Input: part model. Units: mm. Frame: model coordinates. Face numbers are marked on the shaded views. Give positions to 0.01 mm unless a question says otherwise; leave off trailing zeros. Write each loop counter-clockwise with the first axis right and the second up, starting at its lowest first coordinate (ties: lowest second). Pieces come first, ordered by that corner, then holes. Notation, with made-up numbers: (79, 29.25) - (112, 29.25) arc R25 ccw to (112, 42.25) - close; hole circle Ø2 at (-1.5, 19.5). An arc over 180 degrees is marked (long way). Use a Markdown table: item, result. Add a question column.
1. Section query D-D, the plane y = 6. Return loops of the section in (x, z), plus the area to 3 significant figures.
2. Section query B-B, the plane z = 0. Return loops of the section in (x, y), plus the area to 3 significant figures.
3. Mould query, pull axis Z, two halves, no side actions, for the marked faces 1, 2 and 3. Classes: released by +Z, released by -Z, zero draft, split by the parting line, or undercut.
4. Section query C-C, the plane x = 9.5. Return loops of the section in (y, z).
5. Pin query (flat end, axial travel): pin 1 (2 mm diameter, centred on x = -10, y = 8, fed in from -Z); pin 2 (2 mm diameter, centred on x = 2.5, y = 8.5, fed in from -Z); pin 3 (1.5 mm diameter, centred on y = 4, z = 8.5, fed in from -X). Return the tip coordinate at first contact, or that it passes through.
6. Section query A-A, the plane x = 0. Return loops of the section in (y, z), plus the area to 3 significant figures.
7. Material intervals for probe 1 along X at (y, z) = (6.25, 0); probe 2 along X at (y, z) = (8, 1); probe 3 along X at (y, z) = (2.25, 3), sorted ascending.
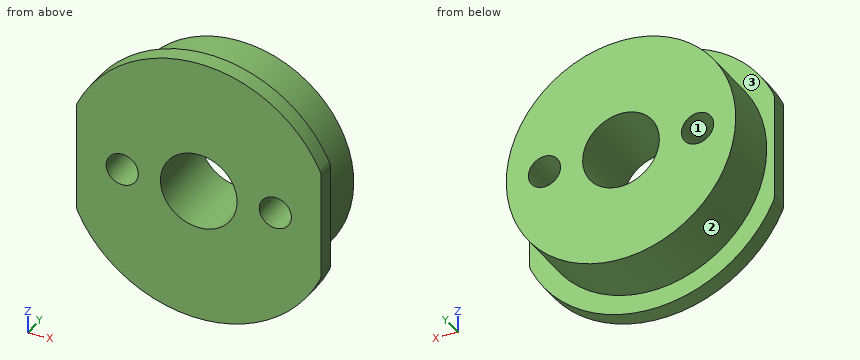
```python
from build123d import *

# Parameters (mm, degrees)
SKETCH_1_R          = 17.5
EXTRUDE_1_DEPTH     = 2.3
SKETCH_2_R          = 14.99
EXTRUDE_2_DEPTH     = 7.7
CUT_EXTRUDE_1_REACH = 28.693
SKETCH_3_R          = 5.01
SKETCH_3_R_2        = 2.1
FILLET_1_R          = 2


with BuildPart() as part:
    # ｽｹｯﾁ1 → ﾎﾞｽ - 押し出し1 (new body)
    with BuildSketch(Plane(origin=(0, 0, 0), x_dir=(1, 0, 0), z_dir=(0, 1, 0))):
        with Locations(Location((0, 0, 0), (0, 0, 270))):
            Circle(SKETCH_1_R)
    extrude(amount=EXTRUDE_1_DEPTH)

    # ｽｹｯﾁ2 → ﾎﾞｽ - 押し出し2 (add)
    with BuildSketch(Plane(origin=(0, 2.3, 0), x_dir=(1, 0, 0), z_dir=(0, 1, 0))):
        with Locations(Location((0, 0, 0), (0, 0, 270))):
            Circle(SKETCH_2_R)
    extrude(amount=EXTRUDE_2_DEPTH)

    # ｶｯﾄ - 押し出し1: up to this face of the body (flat: up to its plane)
    cut_extrude_1_end = Plane(part.part.faces().sort_by_distance((0, 10, 0))[0])
    # ｽｹｯﾁ3 → ｶｯﾄ - 押し出し1 (cut, up to the picked face)
    with BuildSketch(Plane.XZ, mode=Mode.PRIVATE) as cut_extrude_1_sk1:
        with Locations(Location((0, 0, 0), (0, 0, 270))):
            Circle(SKETCH_3_R)
    cut_extrude_1_tool1 = split(extrude(cut_extrude_1_sk1.sketch, amount=-CUT_EXTRUDE_1_REACH, mode=Mode.PRIVATE), bisect_by=cut_extrude_1_end, keep=Keep.BOTH, mode=Mode.PRIVATE)
    # ｽｹｯﾁ3 → ｶｯﾄ - 押し出し1 (cut, up to the picked face)
    with BuildSketch(Plane.XZ, mode=Mode.PRIVATE) as cut_extrude_1_sk2:
        with Locations(Location((10, 0, 0), (0, 0, 270))):
            Circle(SKETCH_3_R_2)
    cut_extrude_1_tool2 = split(extrude(cut_extrude_1_sk2.sketch, amount=-CUT_EXTRUDE_1_REACH, mode=Mode.PRIVATE), bisect_by=cut_extrude_1_end, keep=Keep.BOTH, mode=Mode.PRIVATE)
    # ｽｹｯﾁ3 → ｶｯﾄ - 押し出し1 (cut, up to the picked face)
    with BuildSketch(Plane.XZ, mode=Mode.PRIVATE) as cut_extrude_1_sk3:
        with Locations(Location((-10, 0, 0), (0, 0, 90))):
            Circle(SKETCH_3_R_2)
    cut_extrude_1_tool3 = split(extrude(cut_extrude_1_sk3.sketch, amount=-CUT_EXTRUDE_1_REACH, mode=Mode.PRIVATE), bisect_by=cut_extrude_1_end, keep=Keep.BOTH, mode=Mode.PRIVATE)
    # ｽｹｯﾁ3 → ｶｯﾄ - 押し出し1 (cut, up to the picked face)
    with BuildSketch(Plane.XZ, mode=Mode.PRIVATE) as cut_extrude_1_sk4:
        with BuildLine():
            Line((16, 7.088723439), (16, -7.088723439))
            ThreePointArc((16, -7.088723439), (17.5, 0), (16, 7.088723439))
        make_face()
    cut_extrude_1_tool4 = split(extrude(cut_extrude_1_sk4.sketch, amount=-CUT_EXTRUDE_1_REACH, mode=Mode.PRIVATE), bisect_by=cut_extrude_1_end, keep=Keep.BOTH, mode=Mode.PRIVATE)
    # ｽｹｯﾁ3 → ｶｯﾄ - 押し出し1 (cut, up to the picked face)
    with BuildSketch(Plane.XZ, mode=Mode.PRIVATE) as cut_extrude_1_sk5:
        with BuildLine():
            Line((-16, 7.088723439), (-16, -7.088723439))
            ThreePointArc((-16, -7.088723439), (-17.5, 0), (-16, 7.088723439))
        make_face()
    cut_extrude_1_tool5 = split(extrude(cut_extrude_1_sk5.sketch, amount=-CUT_EXTRUDE_1_REACH, mode=Mode.PRIVATE), bisect_by=cut_extrude_1_end, keep=Keep.BOTH, mode=Mode.PRIVATE)
    add(cut_extrude_1_tool1.solids().sort_by(Axis((0, 0, 0), (0, 1, 0)))[0], mode=Mode.SUBTRACT)
    add(cut_extrude_1_tool2.solids().sort_by(Axis((10, 0, 0), (0, 1, 0)))[0], mode=Mode.SUBTRACT)
    add(cut_extrude_1_tool3.solids().sort_by(Axis((-10, 0, 0), (0, 1, 0)))[0], mode=Mode.SUBTRACT)
    add(cut_extrude_1_tool4.solids().sort_by(Axis((16.60226, 0, 0), (0, 1, 0)))[0], mode=Mode.SUBTRACT)
    add(cut_extrude_1_tool5.solids().sort_by(Axis((-16.60226, 0, 0), (0, 1, 0)))[0], mode=Mode.SUBTRACT)

    # ﾌｨﾚｯﾄ1
    fillet_1_edges = [part.edges().sort_by_distance(p)[0] for p in [
        (-16, 1.15, 7.088723439),
        (-16, 1.15, -7.088723439),
        (16, 1.15, -7.088723439),
        (16, 1.15, 7.088723439),
    ]]
    fillet(fillet_1_edges, radius=FILLET_1_R)


solid = part.part
```
Result sheet:
| question | item | result |
|---|---|---|
| 1 | outline | circle Ø29.98 at (0, 0); hole circle Ø4.2 at (-10, 0); hole circle Ø10.02 at (0, 0); hole circle Ø4.2 at (10, 0) |
| 1 | area | 599 mm² |
| 2 | outline | (-16, 0) - (-12.1, 0) - (-12.1, 10) - (-14.99, 10) - (-14.99, 2.3) - (-16, 2.3) - close; (-7.9, 0) - (-5.01, 0) - (-5.01, 10) - (-7.9, 10) - close; (5.01, 0) - (7.9, 0) - (7.9, 10) - (5.01, 10) - close; (12.1, 0) - (16, 0) - (16, 2.3) - (14.99, 2.3) - (14.99, 10) - (12.1, 10) - close |
| 2 | area | 120 mm² |
| 3 | face 1 | undercut |
| 3 | face 2 | split by the parting line |
| 3 | face 3 | zero draft |
| 4 | outline | (0, -14.7) - (2.3, -14.7) - (2.3, -11.6) - (10, -11.6) - (10, -2.04) - (0, -2.04) - close; (0, 2.04) - (10, 2.04) - (10, 11.6) - (2.3, 11.6) - (2.3, 14.7) - (0, 14.7) - close |
| 5 | pin 1 | stops at z = -11.99 |
| 5 | pin 2 | stops at z = -14.91 |
| 5 | pin 3 | stops at x = -12.83 |
| 6 | outline | (0, -17.5) - (2.3, -17.5) - (2.3, -14.99) - (10, -14.99) - (10, -5.01) - (0, -5.01) - close; (0, 5.01) - (10, 5.01) - (10, 14.99) - (2.3, 14.99) - (2.3, 17.5) - (0, 17.5) - close |
| 6 | area | 211 mm² |
| 7 | probe 1 | x = -14.99 to -12.1, -7.9 to -5.01, 5.01 to 7.9, 12.1 to 14.99 |
| 7 | probe 2 | x = -14.96 to -11.85, -8.15 to -4.91, 4.91 to 8.15, 11.85 to 14.96 |
| 7 | probe 3 | x = -16 to -4.01, 4.01 to 16 |
